The listing builds one solid part. Answer for the finished solid, in the listing's coordinates (mm). A direction names the side the tool comes from. Coordinates: 2 decimals unless noted, no trailing zeros. Order: outer loops, then holes, each group sorted by start corner. A loop starts at its lowest first (then second) coordinate and runs counter-clockwise, first axis right, second up. Notation, with made-up numbers: (49.5, -24.5) - (80.5, -24.5) arc R13 ccw to (80.5, -10.5) - close; hole circle Ø9 at (-38.75, 46.25). An arc over 180 degrees is marked (long way). Use a Markdown table: item, result. Add a question column.
Item 1: For faces 1 (the flat face through (45, -16, 3)), 2 (the cylindrical face through (19.537, -13.935, 4.781)), 3 (the cylindrical face through (11.212, 0.13, 1.232)), determine the directions among +Z, -Z, +X, -X, +Y, -Y from which every point of the face is accessible in a straight line to the end or side of a thin tool.
Item 2: The part is cut by section C-C, the plane y = -61. Give the vertices of the cut face in (x, z), then the cut area to 3 significant figures.
Item 3: Find the intervals of material crossed by line 1 along Y through (x, z) = (26, 5.75); line 2 along Y through (x, z) = (11.5, 0.75); line 3 along X through (y, z) = (-40, 5.25), in increasing order.
Item 4: The part is cut by section A-A, the plane x = -6.5. Give the vertices of the cut face in (y, z), then the cut area to 3 significant figures.
Item 5: The mould has two halves that part along X. Classify faces 4 (the flat face through (34, 1, 7)), 5 (the flat face through (22.4, -42.1, 3)): released by +X, released by -X, zero draft, split by the parting line, or undercut.
Item 6: Flat-ended cylindrical pins translate along their axes: P1, Ø1.1, axis at y = -11.5, z = 1, coming from the +X side; P2, Ø1.5, axis at x = 26, z = 2, coming from the -Y side; P3, Ø2, axis at y = -24, z = 1.5, coming from the -X side. Find the tip coordinate at first contact, or state that the pin passes through.
Item 7: The part is cut by section B-B, the plane x = 19.5. State how many separate pieces and enclosed holes the cut face has, then the cut area to 3 significant figures.
Item 8: The part is cut by section D-D, the plane y = 45.5. Give the vertices of the cut face in (x, z), then the cut area to 3 significant figures.
from build123d import *

# Parameters (mm, degrees)
SKETCH1_R           = 65.5
SKETCH1_R_2         = 1.7
BOSS_EXTRUDE1_DEPTH = 7
BOSS_EXTRUDE2_START = -7
SKETCH2_R           = 70.5
SKETCH2_R_2         = 65.5
BOSS_EXTRUDE2_DEPTH = 7
SKETCH5_R           = 2.7
SKETCH5_R_2         = 2.699999999
SKETCH5_R_3         = 1.5
SKETCH5_R_4         = 1.499999999
CUT_EXTRUDE3_DEPTH  = 15
SKETCH6_R           = 4.500000001
CUT_EXTRUDE4_DEPTH  = 4
BOSS_EXTRUDE3_START = -7
SKETCH8_R           = 1.7
BOSS_EXTRUDE3_DEPTH = 7
SKETCH9_R           = 1.7
CUT_EXTRUDE5_DEPTH  = 14
SKETCH10_R          = 2.95
CUT_EXTRUDE6_DEPTH  = 2.5
SKETCH11_R          = 1.7
CUT_EXTRUDE7_DEPTH  = 9.5
SKETCH12_R          = 2.95
CUT_EXTRUDE8_DEPTH  = 2.5
CUT_EXTRUDE9_START  = -7
CUT_EXTRUDE9_DEPTH  = 4.5
CUT_EXTRUDE11_DEPTH = 2.5
SKETCH15_R          = 4.5
CUT_EXTRUDE12_DEPTH = 4
CUT_EXTRUDE13_DEPTH = 2.5


# Read off the part's stored shape, not the designer's step: Cut-Extrude9
with BuildPart() as part:
    # Sketch1 → Boss-Extrude1 (new body)
    with BuildSketch(Plane.XY):
        with Locations((19.5, 0)):
            Circle(SKETCH1_R)
        with Locations((26.5, 0)):
            Circle(SKETCH1_R_2, mode=Mode.SUBTRACT)
        with Locations((19.5, -7)):
            Circle(SKETCH1_R_2, mode=Mode.SUBTRACT)
        with Locations((12.5, 0)):
            Circle(SKETCH1_R_2, mode=Mode.SUBTRACT)
        with Locations((19.5, 7)):
            Circle(SKETCH1_R_2, mode=Mode.SUBTRACT)
    extrude(amount=BOSS_EXTRUDE1_DEPTH)

    # Sketch2 → Boss-Extrude2 (add)
    with BuildSketch(Plane.XY.offset(7).offset(BOSS_EXTRUDE2_START)):
        with Locations((19.5, 0)):
            Circle(SKETCH2_R)
        with Locations((19.5, 0)):
            Circle(SKETCH2_R_2, mode=Mode.SUBTRACT)
    extrude(amount=BOSS_EXTRUDE2_DEPTH)

    # Sketch5 → Cut-Extrude3 (cut)
    with BuildSketch(Plane(origin=(0, 0, 0), x_dir=(-1, 0, 0), z_dir=(0, 0, -1))):
        with Locations((-45.499999999, -12.898668068)):
            Circle(SKETCH5_R)
        with Locations((6.5, -12.898668066)):
            Circle(SKETCH5_R_2)
        with Locations((-19.499999998, -42.185)):
            Circle(SKETCH5_R_2)
        with Locations((-37.4, 2.264186636)):
            Circle(SKETCH5_R_3)
        with Locations((-37.399999999, -28.061522771)):
            Circle(SKETCH5_R_4)
        with Locations((-1.599999999, -28.06152277)):
            Circle(SKETCH5_R_4)
        with Locations((-1.6, 2.264186638)):
            Circle(SKETCH5_R_3)
    extrude(amount=-CUT_EXTRUDE3_DEPTH, mode=Mode.SUBTRACT)

    # Sketch6 → Cut-Extrude4 (cut)
    with BuildSketch(Plane.XY.offset(7)):
        with Locations((19.499999998, -42.185)):
            Circle(SKETCH6_R)
    extrude(amount=-CUT_EXTRUDE4_DEPTH, mode=Mode.SUBTRACT)

    # Sketch8 → Boss-Extrude3 (add)
    with BuildSketch(Plane.XY.offset(7).offset(BOSS_EXTRUDE3_START)):
        with Locations((12.5, 0)):
            Circle(SKETCH8_R)
        with Locations((19.5, -7)):
            Circle(SKETCH8_R)
        with Locations((26.5, 0)):
            Circle(SKETCH8_R)
        with Locations((19.5, 7)):
            Circle(SKETCH8_R)
    extrude(amount=BOSS_EXTRUDE3_DEPTH)

    # Sketch9 → Cut-Extrude5 (cut)
    with BuildSketch(Plane.XY.offset(7)):
        with Locations((19.5, 11.235)):
            Circle(SKETCH9_R)
        with Locations((27.444344687, 7.944344686)):
            Circle(SKETCH9_R)
        with Locations((30.735, -1e-09)):
            Circle(SKETCH9_R)
        with Locations((27.444344686, -7.944344687)):
            Circle(SKETCH9_R)
        with Locations((19.5, -11.235)):
            Circle(SKETCH9_R)
        with Locations((11.555655313, -7.944344687)):
            Circle(SKETCH9_R)
        with Locations((8.265, 0)):
            Circle(SKETCH9_R)
        with Locations((11.555655314, 7.944344686)):
            Circle(SKETCH9_R)
    extrude(amount=-CUT_EXTRUDE5_DEPTH, mode=Mode.SUBTRACT)

    # Sketch10 → Cut-Extrude6 (cut)
    with BuildSketch(Plane(origin=(0, 0, 0), x_dir=(-1, 0, 0), z_dir=(0, 0, -1))):
        with Locations((-19.5, -11.235)):
            Circle(SKETCH10_R)
        with Locations((-27.444344687, -7.944344687)):
            Circle(SKETCH10_R)
        with Locations((-30.735, 0)):
            Circle(SKETCH10_R)
        with Locations((-27.444344687, 7.944344687)):
            Circle(SKETCH10_R)
        with Locations((-19.5, 11.235)):
            Circle(SKETCH10_R)
        with Locations((-11.555655313, 7.944344687)):
            Circle(SKETCH10_R)
        with Locations((-8.265, 0)):
            Circle(SKETCH10_R)
        with Locations((-11.555655313, -7.944344687)):
            Circle(SKETCH10_R)
    extrude(amount=-CUT_EXTRUDE6_DEPTH, mode=Mode.SUBTRACT)

    # Sketch11 → Cut-Extrude7 (cut)
    with BuildSketch(Plane.XY.offset(7)):
        with Locations((19.5, 0)):
            Circle(SKETCH11_R)
    extrude(amount=-CUT_EXTRUDE7_DEPTH, mode=Mode.SUBTRACT)

    # Sketch12 → Cut-Extrude8 (cut)
    with BuildSketch(Plane(origin=(0, 0, 0), x_dir=(-1, 0, 0), z_dir=(0, 0, -1))):
        with Locations((-19.5, 0)):
            Circle(SKETCH12_R)
    extrude(amount=-CUT_EXTRUDE8_DEPTH, mode=Mode.SUBTRACT)

    # Cut-Extrude9 outline → Cut-Extrude9 (cut)
    with BuildSketch(Plane(origin=(0, 0, 0), x_dir=(-1, 0, 0), z_dir=(0, 0, -1)).offset(CUT_EXTRUDE9_START)):
        with BuildLine():
            Line((-21.2, -11.235), (-21.199999984, -12.235))
            ThreePointArc((-21.199999984, -12.235), (-19.499999992, -13.934999993), (-17.8, -12.235))
            Line((-17.8, -12.235), (-17.8, -11.235))
            ThreePointArc((-17.8, -11.235), (-19.5, -12.935), (-21.2, -11.235))
        make_face()
        with BuildLine():
            Line((-21.2, 12.235), (-21.2, 11.235))
            ThreePointArc((-21.2, 11.235), (-19.5, 12.935), (-17.8, 11.235))
            Line((-17.8, 11.235), (-17.8, 12.235))
            ThreePointArc((-17.8, 12.235), (-19.5, 13.935), (-21.2, 12.235))
        make_face()
    extrude(amount=CUT_EXTRUDE9_DEPTH, mode=Mode.SUBTRACT)

    # Sketch14 → Cut-Extrude11 (cut)
    with BuildSketch(Plane(origin=(0, 0, 0), x_dir=(-1, 0, 0), z_dir=(0, 0, -1))):
        with BuildLine():
            Line((-22.45, 11.235), (-22.45, 12.235))
            ThreePointArc((-22.45, 12.235), (-19.5, 15.185), (-16.55, 12.235))
            Line((-16.55, 12.235), (-16.55, 11.235))
            ThreePointArc((-16.55, 11.235), (-19.5, 8.285), (-22.45, 11.235))
        make_face()
        with BuildLine():
            Line((-16.549999992, -11.235), (-16.549999992, -12.235))
            ThreePointArc((-16.549999992, -12.235), (-19.499999992, -15.185000015), (-22.450000007, -12.235))
            Line((-22.450000007, -12.235), (-22.450000007, -11.235))
            ThreePointArc((-22.450000007, -11.235), (-19.5, -8.284999993), (-16.549999992, -11.235))
        make_face()
    extrude(amount=-CUT_EXTRUDE11_DEPTH, mode=Mode.SUBTRACT)

    # Sketch15 → Cut-Extrude12 (cut)
    with BuildSketch(Plane.XY.offset(7)):
        with Locations((45.499999999, -12.898668068)):
            Circle(SKETCH15_R)
        with Locations((-6.5, -12.898668066)):
            Circle(SKETCH15_R)
    extrude(amount=-CUT_EXTRUDE12_DEPTH, mode=Mode.SUBTRACT)

    # Sketch16 → Cut-Extrude13 (cut)
    with BuildSketch(Plane(origin=(0, 0, 0), x_dir=(-1, 0, 0), z_dir=(0, 0, -1))):
        with BuildLine():
            Line((-22.7, 11.235), (-22.7, 12.235))
            ThreePointArc((-22.7, 12.235), (-19.5, 15.435), (-16.3, 12.235))
            Line((-16.3, 12.235), (-16.3, 11.235))
            ThreePointArc((-16.3, 11.235), (-19.5, 8.035), (-22.7, 11.235))
        make_face()
        with BuildLine():
            Line((-16.3, -11.235), (-16.3, -12.235))
            ThreePointArc((-16.3, -12.235), (-19.499999992, -15.435000008), (-22.7, -12.235))
            Line((-22.7, -12.235), (-22.7, -11.235))
            ThreePointArc((-22.7, -11.235), (-19.5, -8.035), (-16.3, -11.235))
        make_face()
    extrude(amount=-CUT_EXTRUDE13_DEPTH, mode=Mode.SUBTRACT)


solid = part.part
Solution:
| question | item | result |
|---|---|---|
| 1 | face 1 | +Z |
| 1 | face 2 | +Z, -Z |
| 1 | face 3 | -Z |
| 2 | outline | (-15.84, 0) - (54.84, 0) - (54.84, 7) - (-15.84, 7) - close |
| 2 | area | 495 mm2 |
| 3 | line 1 | y = -70.2 to -8.84, -7.05 to 7.05, 8.84 to 70.2 |
| 3 | line 2 | y = -70.04 to -10.89, -4.99 to 4.99, 10.89 to 70.04 |
| 3 | line 3 | x = -38.55 to 15.57, 23.43 to 77.55 |
| 4 | outline | (-65.53, 0) - (-15.6, 0) - (-15.6, 3) - (-17.4, 3) - (-17.4, 7) - (-65.53, 7) - close; (-10.2, 0) - (65.53, 0) - (65.53, 7) - (-8.4, 7) - (-8.4, 3) - (-10.2, 3) - close |
| 4 | area | 865 mm2 |
| 5 | face 4 | zero draft |
| 5 | face 5 | undercut |
| 6 | P1 | stops at x = 89.14 |
| 6 | P2 | stops at y = -70.27 |
| 6 | P3 | stops at x = -47.14 |
| 7 | separate pieces | 5 |
| 7 | enclosed holes | 0 |
| 7 | area | 828 mm2 |
| 8 | outline | (-34.35, 0) - (73.35, 0) - (73.35, 7) - (-34.35, 7) - close |
| 8 | area | 754 mm2 |
